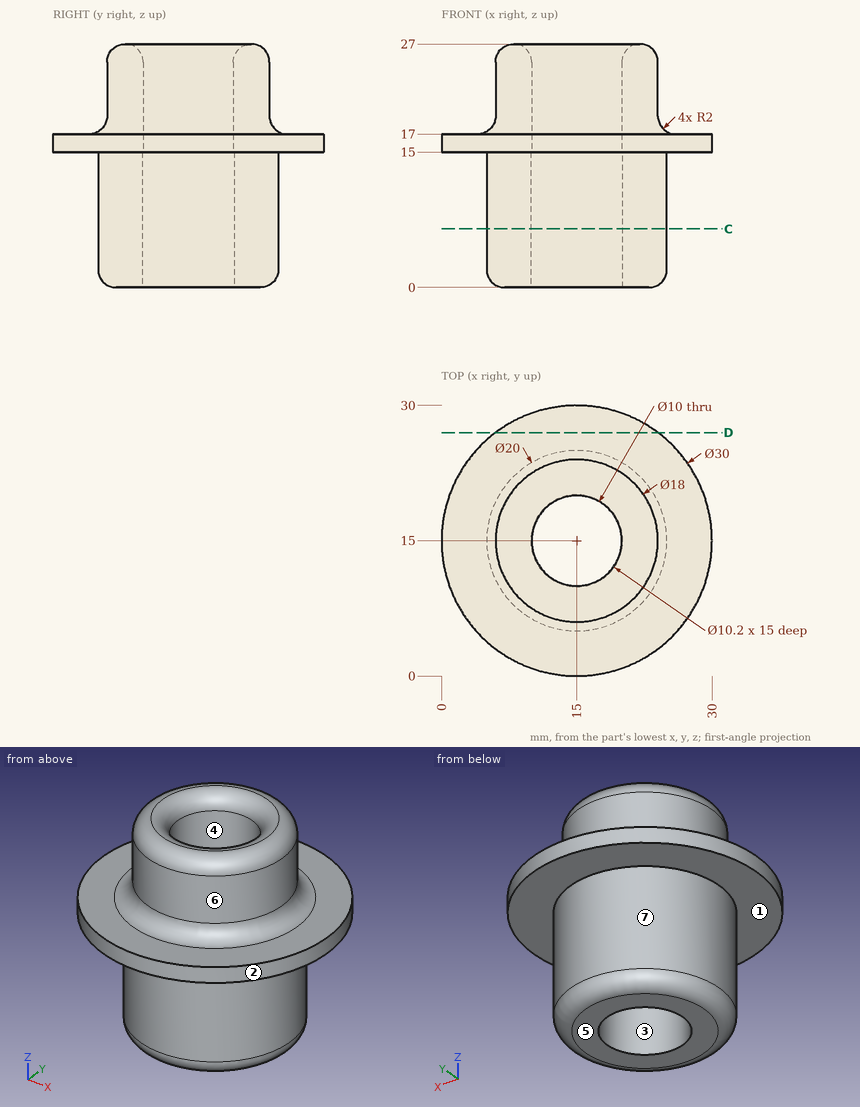
Design review of the part shown in the three views and the two pictorial views. Dimensions are in mm from the part's minimum x, y and z. A direction names the side the tool comes from. Round coordinates to 2 decimals unless told otherwise and drop trailing zeros. Write each loop counter-clockwise with the first axis right and the second up, starting at its lowest first coordinate (ties: lowest second). Pieces come first, ordered by that corner, then holes. Notation, with made-up numbers: M 45,82 L 94,82 A30 ccw 94,109 Z; hole C -1.75,89.5 d3. An arc over 180 degrees is marked long. Use a Markdown table: item, result. Add a question column.
Q1. To check wall thickness, follow line 1 (Y direction, x = 15, z = 20.5); line 2 (Y direction, x = 15, z = 9.25); line 3 (Z direction, x = 10.5, y = 27.25). State the ranges of each line that lie inside material, in increasing order.
Q2. Insertion check: pin 1 (13 mm diameter, centred on x = 15, y = 15, fed in from +Z); pin 2 (1.5 mm diameter, centred on y = 26, z = 17, fed in from -X); pin 3 (3 mm diameter, centred on x = 6.5, z = 14, fed in from +Y). Each pin has a flat end and moves straight along its axis. Give the tip position at first contact, or say it passes through.
Q3. Machinability: for the marked faces 5, 6 and 7, which of the approach directions +Z, -Z, +X, -X, +Y, -Y give a long, thin tool a straight path to every point of the face, cutting with its end or side? Answer none if there is none.
Q4. We need section C-C, the plane z = 6.5. State the section outline as (x, y) points.
Q5. We need section D-D, the plane y = 27. State the section outline as (x, z) points.
Q6. The part is to be moulded in two halves that separate along Y. For the marked faces 1, 2, 3 and 4, say which applies: pulls with the +Y half, pulls with the -Y half, needs draft (parallel to the pull), parting line crosses it, or undercut.
Findings below:
| question | item | result |
|---|---|---|
| 1 | line 1 | y = 6 to 10, 20 to 24 |
| 1 | line 2 | y = 5 to 9.9, 20.1 to 25 |
| 1 | line 3 | z = 15 to 17 |
| 2 | pin 1 | stops at z = 26.94 |
| 2 | pin 2 | stops at x = 4.05 |
| 2 | pin 3 | stops at y = 28.06 |
| 3 | face 5 | -Z, +X, -X, +Y, -Y |
| 3 | face 6 | +Z |
| 3 | face 7 | -Z |
| 4 | outline | C 15,15 d20; hole C 15,15 d10.2 |
| 5 | outline | M 6,15 L 24,15 L 24,17 L 6,17 Z |
| 6 | face 1 | needs draft |
| 6 | face 2 | parting line crosses it |
| 6 | face 3 | undercut |
| 6 | face 4 | undercut |
